```python
from build123d import *

# Parameters (mm, degrees)
CROQUIS1_W              = 650
CROQUIS1_H              = 550
SALIENTE_EXTRUIR1_DEPTH = 28
VACIADO1_T              = -2
CROQUIS2_W              = 646
CROQUIS2_H              = 2
SALIENTE_EXTRUIR2_DEPTH = 10
CROQUIS3_W              = 646
CROQUIS3_H              = 2
SALIENTE_EXTRUIR3_DEPTH = 10
CORTAR_EXTRUIR1_REACH   = 708.335
CROQUIS4_W              = 15
CROQUIS4_H              = 5


with BuildPart() as part:
    # Croquis1 → Saliente-Extruir1 (new body)
    with BuildSketch(Plane(origin=(0, 0, 0), x_dir=(1, 0, 0), z_dir=(0, 1, 0))):
        Rectangle(CROQUIS1_W, CROQUIS1_H)
    extrude(amount=SALIENTE_EXTRUIR1_DEPTH)

    # Vaciado1
    vaciado1_openings = [part.faces().sort_by_distance(p)[0] for p in [
        (0, 0, 0),
    ]]
    offset(amount=VACIADO1_T, openings=vaciado1_openings, kind=Kind.INTERSECTION)

    # Croquis2 → Saliente-Extruir2 (add)
    with BuildSketch(Plane(origin=(0, 0, 273), x_dir=(-1, 0, 0), z_dir=(0, 0, -1))):
        with Locations((0, 1)):
            Rectangle(CROQUIS2_W, CROQUIS2_H)
    extrude(amount=SALIENTE_EXTRUIR2_DEPTH)

    # Croquis3 → Saliente-Extruir3 (add)
    with BuildSketch(Plane.XY.offset(-273)):
        with Locations((0, 1)):
            Rectangle(CROQUIS3_W, CROQUIS3_H)
    extrude(amount=SALIENTE_EXTRUIR3_DEPTH)

    # Cortar-Extruir1: up to this face of the body (flat: up to its plane)
    cortar_extruir1_end = Plane(part.part.faces().sort_by_distance((325, 14, 0))[0])
    # Croquis4 → Cortar-Extruir1 (cut, up to the picked face)
    with BuildSketch(Plane.ZY.offset(325), mode=Mode.PRIVATE) as cortar_extruir1_sk1:
        with Locations((-247.5, 14)):
            Rectangle(CROQUIS4_W, CROQUIS4_H)
    cortar_extruir1_tool1 = split(extrude(cortar_extruir1_sk1.sketch, amount=-CORTAR_EXTRUIR1_REACH, mode=Mode.PRIVATE), bisect_by=cortar_extruir1_end, keep=Keep.BOTH, mode=Mode.PRIVATE)
    # Croquis4 → Cortar-Extruir1 (cut, up to the picked face)
    with BuildSketch(Plane.ZY.offset(325), mode=Mode.PRIVATE) as cortar_extruir1_sk2:
        with Locations((247.5, 14)):
            Rectangle(CROQUIS4_W, CROQUIS4_H)
    cortar_extruir1_tool2 = split(extrude(cortar_extruir1_sk2.sketch, amount=-CORTAR_EXTRUIR1_REACH, mode=Mode.PRIVATE), bisect_by=cortar_extruir1_end, keep=Keep.BOTH, mode=Mode.PRIVATE)
    add(cortar_extruir1_tool1.solids().sort_by(Axis((-325, 14, -247.5), (1, 0, 0)))[0], mode=Mode.SUBTRACT)
    add(cortar_extruir1_tool2.solids().sort_by(Axis((-325, 14, 247.5), (1, 0, 0)))[0], mode=Mode.SUBTRACT)


solid = part.part
```
The model under review builds one solid part; all positions refer to its coordinate system, in mm. Round coordinates to 2 decimals unless told otherwise and drop trailing zeros. Loops run counter-clockwise (first coordinate to the right, second up) from the corner with the lowest first, then second, coordinate; pieces in that order, holes last.
Item 1: Mouldability with a two-part tool opening along Y and no side actions: class faces 1 (the face through (-5, 28, -4)), 2 (the face through (-325, 14, 4)), 3 (the face through (-5, 14, 273)), 4 (the face through (-5, 14, -273)) as released by +Y, released by -Y, zero draft, split by the parting line, or undercut.
Determined:
face 1: released by +Y
face 2: zero draft
face 3: undercut
face 4: undercut
Item 2: Take a section at C-C (x = -27). Write out the cut boundary in (y, z), then the cut area to 3 significant figures.
Determined:
outline: (0, -275) - (28, -275) - (28, 275) - (0, 275) - (0, 263) - (2, 263) - (2, 273) - (26, 273) - (26, -273) - (2, -273) - (2, -263) - (0, -263) - close
area: 1,240 mm2
Item 3: Take a section at B-B (z = 56). Write out the cut boundary in (x, y), then the cut area to 3 significant figures.
Determined:
outline: (-325, 0) - (-323, 0) - (-323, 26) - (323, 26) - (323, 0) - (325, 0) - (325, 28) - (-325, 28) - close
area: 1,400 mm2
Item 4: For line 1 (X direction, y = 2, z = 55); line 2 (Z direction, x = -120.5, y = 18.5); line 3 (Z direction, x = 162, y = 1.5), list the stretches that pass through material, from the lowest coordinate up.
Determined:
line 1: x = -325 to -323, 323 to 325
line 2: z = -275 to -273, 273 to 275
line 3: z = -275 to -263, 263 to 275
Item 5: Clearance check with flat-ended pins moving along their axes: pin 1 Ø1.6 at (x, z) = (-323.5, 248.5) entering from -Y; pin 2 Ø2 at (x, z) = (214, 22) entering from -Y. State where each tip first meets the part, or that it passes through.
Determined:
pin 1: stops at y = 0
pin 2: stops at y = 26
Item 6: Take a section at A-A (y = 7). Write out the cut boundary in (x, z), then the cut area to 3 significant figures.
Determined:
outline: (-325, -275) - (325, -275) - (325, 275) - (-325, 275) - close; hole (-323, -273) - (323, -273) - (323, 273) - (-323, 273) - close
area: 4,780 mm2
